Autodesk Inventor part; units mm, degrees
ref_plane "YZ Plane" through (0, 0, 0) normal (1, 0, 0) x (0, 1, 0)
ref_plane "XZ Plane" through (0, 0, 0) normal (0, 1, 0) x (-1, 0, 0)
ref_plane "XY Plane" through (0, 0, 0) normal (0, 0, 1) x (1, 0, 0)
sketch "스케치1" plane through (0, 0, 0) normal (0, 0, 1) x (1, 0, 0)
  circle A0 centre (0, 0) radius 31.5
  dimension "d0" = 63
extrude "돌출1" add sketch "스케치1" along normal blind 27.5
sketch "스케치2" plane through (0, 0, 27.5) normal (0, 0, 1) x (1, 0, 0)
  circle A0 centre (0, 0) radius 26.5
  dimension "d3" = 53
extrude "돌출2" add sketch "스케치2" along normal blind 5
sketch "스케치3" plane through (0, 0, 0) normal (0, 0, -1) x (-1, 0, 0)
  circle A0 centre (0, 0) radius 26.5
  circle A1 centre (0, 0) radius 26.5
  dimension "d6" = 53
extrude "돌출3" add sketch "스케치3" along normal blind 9
sketch "스케치5" plane through (0, 0, 32.5) normal (0, 0, 1) x (1, 0, 0)
  circle A0 centre (0, 0) radius 13.5
  circle A1 centre (-6.75, 11.6913) radius 1.5
  circle A2 centre (-6.75, -11.6913) radius 1.5
  circle A3 centre (13.5, 0) radius 1.5
  dimension "d19" = 360
  dimension "d39" = 360
  dimension "d13" = 27
  dimension "d43" = 360
extrude "돌출5" cut sketch "스케치5" against normal blind 3 contours A0 A3 | A0 A3 | A1 A0 | A0 A1 | A2 A0 | A0 A2
sketch "스케치6" plane through (0, 0, -9) normal (0, 0, -1) x (-1, 0, 0)
  circle A0 centre (0, 0) radius 24
  circle A1 centre (24, 0) radius 1.5
  circle A2 centre (12, 20.7846) radius 1.5
  circle A3 centre (-12, 20.7846) radius 1.5
  circle A4 centre (-24, 0) radius 1.5
  circle A5 centre (-12, -20.7846) radius 1.5
  circle A6 centre (12, -20.7846) radius 1.5
  dimension "d21" = 48
  dimension "d22" = 3
  dimension "d25" = 360
extrude "돌출6" cut sketch "스케치6" against normal blind 8 contours A0 A1 | A0 A1 | A2 A0 | A0 A2 | A6 A0 | A0 A6 | A3 A0 | A0 A3 | A5 A0 | A0 A5 | A4 A0 | A0 A4
sketch "스케치7" plane through (0, 0, 0) normal (0, 0, -1) x (-1, 0, 0)
  circle A0 centre (0, 0) radius 29
  circle A1 centre (-29, 0) radius 1.25
  circle A2 centre (-14.5, -25.1147) radius 1.25
  circle A3 centre (14.5, -25.1147) radius 1.25
  circle A4 centre (29, 0) radius 1.25
  circle A5 centre (14.5, 25.1147) radius 1.25
  circle A6 centre (-14.5, 25.1147) radius 1.25
  dimension "d29" = 58
  dimension "d30" = 2.5
  dimension "d33" = 360
extrude "돌출7" cut sketch "스케치7" against normal blind 53.25 contours A0 A4 | A0 A4 | A5 A0 | A0 A5 | A3 A0 | A0 A3 | A6 A0 | A0 A6 | A2 A0 | A0 A2 | A1 A0 | A0 A1
properties part number "부품1"
Model file for the job. Use its own axes, mm. A direction names the side the tool comes from. Coordinates: 2 decimals unless noted, no trailing zeros. Loops run counter-clockwise (first coordinate to the right, second up) from the corner with the lowest first, then second, coordinate; pieces in that order, holes last. Notation, with made-up numbers: (51.5, 59.25) - (99.5, 59.25) arc R17 ccw to (99.5, 67.25) - close; hole circle Ø3 at (61, 11.25). An arc over 180 degrees is marked (long way). Answer as a JSON object with one key per item and string values. Group by question number.
(1) Tool access for faces 5 (the face through (-13.58, 25.96, 13.56)), 6 (the face through (13, 0, 29.5)), 7 (the face through (12, -21, -1)): list every direction of +Z, -Z, +X, -X, +Y, -Y with a clear straight run to the whole face (end or side of a thin tool).
(2) Cut at B-B (z = -5). Give the cut face in (x, y).
(3) Cut at A-A (x = -29). Give the cut face in (y, z).
(4) Flat gauge pins, fed straight in: pin 1 (4 mm diameter, centred on y = 19, z = 7, fed in from -X); pin 2 (12 mm diameter, centred on x = -19, z = 2.5, fed in from +Y); pin 3 (4 mm diameter, centred on x = -6.75, y = -11.69, fed in from +Z); pin 4 (8 mm diameter, centred on x = -10, z = 25.5, fed in from -Y). Where does each tip first touch, or does it go through?
(5) Two-plate mould, pull along X, no slides. Class faces 1 (the face through (-19, 19, 0)), 2 (the face through (14.246, -22.345, 29.965)), 3 (the face through (-7, -12, 29.5)), 4 (the face through (-30.155, -0.479, 13.558)): released by +X, released by -X, zero draft, split by the parting line, or undercut.
(6) Cut at C-C (y = -5.5). Give the cut face in (x, z).
(7) Probe line 1 along Y through (x, z) = (-6.75, 30.45); line 2 along Y through (x, z) = (-14, 6); line 3 along X through (y, z) = (26, 15). List the from-to ranges inside material, lowest first.
(8) Cut at D-D (x = 0). Give the cut face in (y, z), then the cut area to 3 significant figures.
Geometry says:
{
 "1": {"face 5": "+Z, -Z", "face 6": "+Z", "face 7": "-Z"},
 "2": {"outline": "circle Ø53 at (0, 0); hole circle Ø3 at (-24, 0); hole circle Ø3 at (-12, -20.78); hole circle Ø3 at (-12, 20.78); hole circle Ø3 at (12, -20.78); hole circle Ø3 at (12, 20.78); hole circle Ø3 at (24, 0)"},
 "3": {"outline": "(-12.3, 0) - (-1.25, 0) - (-1.25, 27.5) - (-12.3, 27.5) - close; (1.25, 0) - (12.3, 0) - (12.3, 27.5) - (1.25, 27.5) - close"},
 "4": {"pin 1": "stops at x = -26.52", "pin 2": "stops at y = 28.69", "pin 3": "stops at z = 32.5", "pin 4": "stops at y = -30.92"},
 "5": {"face 1": "zero draft", "face 2": "split by the parting line", "face 3": "undercut", "face 4": "undercut"},
 "6": {"outline": "(-31.02, 0) - (-25.92, 0) - (-25.92, -9) - (25.92, -9) - (25.92, 0) - (31.02, 0) - (31.02, 27.5) - (25.92, 27.5) - (25.92, 32.5) - (-25.92, 32.5) - (-25.92, 27.5) - (-31.02, 27.5) - close"},
 "7": {"line 1": "y = -25.63 to -13.19, -10.19 to 10.19, 13.19 to 25.63", "line 2": "y = -28.22 to -26.26, -23.97 to 23.97, 26.26 to 28.22", "line 3": "x = -17.78 to -15.38, -13.62 to 13.62, 15.38 to 17.78"},
 "8": {"outline": "(-31.5, 0) - (-26.5, 0) - (-26.5, -9) - (26.5, -9) - (26.5, 0) - (31.5, 0) - (31.5, 27.5) - (26.5, 27.5) - (26.5, 32.5) - (-26.5, 32.5) - (-26.5, 27.5) - (-31.5, 27.5) - close", "area": "2,470 mm^2"}
}
